Input: part model. Units: mm. Frame: model coordinates. A direction names the side the tool comes from. Coordinates: 2 decimals unless noted, no trailing zeros. Write each loop counter-clockwise with the first axis right and the second up, starting at its lowest first coordinate (ties: lowest second). Pieces come first, ordered by that corner, then holes. Notation, with made-up numbers: (4, 78) - (10, 78) arc R20 ccw to (10, 105) - close; hole circle Ø6 at (65.5, 64.5). An arc over 180 degrees is marked (long way). Put each result on its own line as item: value. Start each with the question number.
1. Pin query (flat end, axial travel): pin 1 (3 mm diameter, centred on x = 182.5, y = -25, fed in from -Z); pin 2 (1 mm diameter, centred on y = -125.5, z = 43.5, fed in from +X); pin 3 (12 mm diameter, centred on x = 95.5, y = -46.5, fed in from -Z). Return the tip coordinate at first contact, or that it passes through.
2. Cut plane D-D, the plane y = -16. Return loops of the section in (x, z), and give its area (3 significant figures).
3. Pull-direction query (Z, two-part tool) for faces 1 (the flat face through (291.702, -107.929, 3.838)), 2 (the flat face through (18.51, -71.41, 71.51)), 3 (the flat face through (147.902, -72.366, 71.234)); classes: released by +Z, released by -Z, zero draft, split by the parting line, or undercut.
4. Line query: line 1 (Z direction, x = 237, y = -127); line 2 (X direction, y = -126, z = -64); line 3 (X direction, y = -133.5, z = -98.5). Output: solid intervals per line, ascending.
5. Cut plane C-C, the plane z = -11. Return loops of the section in (x, y).
6. Cut plane A-A, the plane y = -73. Return loops of the section in (x, z) (1 decimal), and give its area (3 significant figures).
7. Cut plane B-B, the plane x = 151. Return loops of the section in (y, z), and give its area (3 significant figures).
8. Access query for faces 4 (the flat face through (291.115, -108.828, 3.83)), 5 (the flat face through (8.3, -107.93, -3.84)). Directions: +Z, -Z, +X, -X, +Y, -Y. A direction counts if a zero-diameter tool reaches every point of the face in a straight line with its end or side. Return the directions, or none.
Autodesk Inventor part; units mm, degrees
ref_plane "YZ Plane" through (0, 0, 0) normal (1, 0, 0) x (0, 1, 0)
ref_plane "XZ Plane" through (0, 0, 0) normal (0, 1, 0) x (-1, 0, 0)
ref_plane "XY Plane" through (0, 0, 0) normal (0, 0, 1) x (1, 0, 0)
sketch "Sketch1" plane through (0, 0, 0) normal (1, 0, 0) x (0, 1, 0)
  line L0 (-141.4214, 141.4214) -> (-3.5355, 3.5355)
  line L1 (-141.4214, 141.4214) -> (53.5786, 141.4214) construction
  line L2 (-3.5355, -3.5355) -> (-141.4214, -141.4214)
  line L3 (-141.987, -140.8557) -> (-4.6669, -3.5355)
  line L4 (-4.6669, 3.5355) -> (-141.987, 140.8557)
  line L5 (-141.4214, 141.4214) -> (-141.987, 140.8557)
  line L6 (-141.4214, -141.4214) -> (-141.987, -140.8557)
  arc A0 (-4.6669, -3.5355) -> (-4.6669, 3.5355) centre (-8.2024, 0) ccw
  arc A1 (-3.5355, -3.5355) -> (-3.5355, 3.5355) centre (-7.0711, 0) ccw
  point P0 (0, 0)
  point P1 (0, 0)
  point P2 (-1.1314, 0)
  dimension "d0" = 45
  dimension "d1" = 200
  dimension "d2" = 0.8
  dimension "d3" = 0.8
  dimension "d4" = 200
  dimension "d7" = 5
extrude "Extrusion1" add sketch "Sketch1" along normal blind 300
sketch "Sketch4" plane through (0, 0, 0) normal (0, 0, 1) x (1, 0, 0)
  line L0 (0, -141.4214) -> (0, -3.5355)
  line L1 (0, -141.4214) -> (300, -141.4214)
  line L2 (300, -3.5355) -> (300, -141.4214)
  line L3 (0, -3.5355) -> (300, -3.5355)
  line L4 (300, -4.6669) -> (300, -141.987)
  line L5 (300, -141.987) -> (261.9547, 0)
  line L6 (300, -141.987) -> (444.3601, -141.987) construction
  line L7 (0, -141.987) -> (145.1381, -141.987) construction
  line L8 (300, -2.5459) -> (300, -141.987)
  line L9 (261.9547, 0) -> (300, 0)
  line L10 (300, -3.5355) -> (300, -141.4214)
  line L11 (300, 0) -> (300, -3.5355)
  point P0 (0, 0)
  point P1 (262.6369, -2.5459)
  dimension "d10" = 105
extrude "Extrusion2" cut sketch "Sketch4" along normal through all both and the other way through all contours L5 L3 L2 L1 | L1 L4 L5 | L5 L9 L11 L8 L3
sketch "Sketch5" plane through (299.8484, -141.4214, -141.4214) normal (0.9659258, 0.258819, 0) x (-0.1798136, 0.6710737, -0.7192546)
  line L0 (-203.4359, 195.6898) -> (-203.4359, 196.504)
  line L1 (-5.8996, 202.5394) -> (-203.4359, 195.6898)
  ellipse E0 centre (-5.8996, 197.4504) end of major axis (-2.3034, 201.1736) minor radius 5 (-0.8137, 197.6268) -> (-5.8996, 202.5394) ccw
  line L2 (-0.8137, -0.0282) -> (-0.8137, 197.6268)
  line L3 (0, 0) -> (-0.8137, -0.0282)
  line L4 (0, 198.4692) -> (0, 0)
  ellipse E1 centre (-5.0859, 198.2929) end of major axis (-8.6822, 194.5697) minor radius 5 (0, 198.4692) -> (-5.0859, 203.3818) ccw
  line L5 (-203.4359, 196.504) -> (-5.0859, 203.3818)
  line L6 (-0.8137, -0.0282) -> (-203.4359, 195.6898)
  point P0 (47.103, 252.3228)
extrude "Extrusion3" add sketch "Sketch5" along normal blind 0.8
sketch "Sketch7" plane through (0, 0, 0) normal (0, 0, 1) x (1, 0, 0)
  line L0 (0, -142) -> (38.0488, 0)
  line L1 (0, -142) -> (147.0092, -142) construction
  line L2 (38.0488, 0) -> (0, 0)
  line L3 (0, -3.5355) -> (262.902, -3.5355)
  line L4 (0, 0) -> (0, -142)
  dimension "d18" = 75
extrude "Extrusion4" cut sketch "Sketch7" along normal through all both and the other way through all
sketch "Sketch8" plane through (0.155, -141.4214, 141.4214) normal (-0.9659258, 0.258819, 0) x (0.1798136, 0.6710737, 0.7192546)
  ellipse E0 centre (-5.8996, 197.4504) end of major axis (-2.3034, 201.1736) minor radius 5 (-0.8137, 197.6268) -> (-5.8996, 202.5394) ccw
  line L0 (-0.8137, -0.0282) -> (-0.8137, 197.6268)
  line L1 (0, 0) -> (-0.8137, -0.0282)
  line L2 (0, 198.4692) -> (0, 0)
  ellipse E1 centre (-5.0859, 198.2929) end of major axis (-8.6822, 194.5697) minor radius 5 (0, 198.4692) -> (-5.0859, 203.3818) ccw
  line L3 (-203.4359, 196.504) -> (-5.0859, 203.3818)
  line L4 (-203.4359, 195.6898) -> (-203.4359, 196.504)
  line L5 (-5.8996, 202.5394) -> (-203.4359, 195.6898)
  line L6 (-0.8137, -0.0282) -> (53.1297, 55.8182)
  line L7 (-5.8996, 202.5394) -> (-203.4359, 195.6898)
  line L8 (-0.8137, -0.0282) -> (-203.4359, 195.6898)
  point P0 (-6.8417, 196.4751)
extrude "Extrusion5" add sketch "Sketch8" along normal blind 0.8
equation "\"BendRadius\" = Thickness"
equation "\"BendReliefWidth\" = Thickness"
equation "\"BendReliefDepth\" = 0.5 * Thickness"
equation "\"CornerReliefSize\" = 4 * Thickness"
equation "\"MinimumRemnant\" = 2 * Thickness"
equation "\"TransitionRadius\" = BendRadius"
equation "\"JacobiRadiusSize\" = Thickness"
equation "\"GapSize\" = Thickness"
properties part number "chimneyRoof"
Report:
1. pin 1: stops at z = -26.5
1. pin 2: stops at x = 296.54
1. pin 3: stops at z = -52.5
2. outline: (32.93, -16.21) - (33.76, -16) - (266.24, -16) - (267.07, -16.21) - (267.07, 16.21) - (266.24, 16) - (33.76, 16) - (32.93, 16.21) - close; hole (33.76, -14.87) - (266.24, -14.87) - (266.24, 14.87) - (33.76, 14.87) - close
2. area: 579 mm^2
3. face 1: zero draft
3. face 2: released by +Z
3. face 3: undercut
4. line 1: z = -127 to -125.87, 125.87 to 127
4. line 2: x = 3.46 to 4.29, 295.72 to 296.54
4. line 3: x = 1.45 to 2.28, 297.73 to 298.55
5. outline: (-0.77, -141.78) - (0, -141.99) - (34.8, -12.13) - (265.21, -12.13) - (300, -141.99) - (300.77, -141.78) - (265.67, -10.79) - (264.9, -11) - (35.1, -11) - (34.33, -10.79) - close
6. outline: (17.7, -73.2) - (18.5, -73) - (281.5, -73) - (282.3, -73.2) - (282.3, 73.2) - (281.5, 73) - (18.5, 73) - (17.7, 73.2) - close; hole (18.5, -71.9) - (281.5, -71.9) - (281.5, 71.9) - (18.5, 71.9) - close
6. area: 837 mm^2
7. outline: (-141.99, -140.86) - (-141.42, -141.42) - (-3.54, -3.54) arc R5 ccw to (-3.54, 3.54) - (-141.42, 141.42) - (-141.99, 140.86) - (-4.67, 3.54) arc R5 cw to (-4.67, -3.54) - close
7. area: 319 mm^2
8. face 4: -Y
8. face 5: +Z, -Z, -X, +Y
